from build123d import *

# Parameters (mm, degrees)
SKETCH1_W           = 300
SKETCH1_H           = 50
BOSS_EXTRUDE1_DEPTH = 6
SKETCH2_W           = 220
SKETCH2_H           = 25
CUT_EXTRUDE1_DEPTH  = 10
FILLET1_R           = 10


with BuildPart() as part:
    # Sketch1 → Boss-Extrude1 (new body)
    with BuildSketch(Plane(origin=(0, 0, 0), x_dir=(0, 0, -1), z_dir=(1, 0, 0))):
        Rectangle(SKETCH1_W, SKETCH1_H)
    extrude(amount=BOSS_EXTRUDE1_DEPTH)

    # Sketch2 → Cut-Extrude1 (cut)
    with BuildSketch(Plane(origin=(6, 0, 0), x_dir=(0, 0, -1), z_dir=(1, 0, 0))):
        with Locations((0, -12.5)):
            Rectangle(SKETCH2_W, SKETCH2_H)
    extrude(amount=-CUT_EXTRUDE1_DEPTH, mode=Mode.SUBTRACT)

    # Fillet1
    fillet1_edges = [part.edges().sort_by_distance(p)[0] for p in [
        (3, 0, 110),
        (3, 0, -110),
    ]]
    fillet(fillet1_edges, radius=FILLET1_R)


solid = part.part
Input: part model. Units: mm. Frame: model coordinates. A direction names the side the tool comes from. Coordinates: 2 decimals unless noted, no trailing zeros. Loops run counter-clockwise (first coordinate to the right, second up) from the corner with the lowest first, then second, coordinate; pieces in that order, holes last. Notation, with made-up numbers: (73, 41) -> (78, 41) arc R33 ccw to (78, 70) -> close; hole circle Ø10 at (-27.75, -35). An arc over 180 degrees is marked (long way). One line per item, written item: value.
(1) Draft query along Z for faces 1 (the face through (6, 6, 2)), 2 (the face through (3, 0, 150)), 3 (the face through (2.96, -3.01, -107.15)), 4 (the face through (3, 0, 1)). Return one class per face: pulls with the +Z half, pulls with the -Z half, needs draft (parallel to the pull), parting line crosses it, or undercut.
Answer below:
face 1: needs draft
face 2: pulls with the +Z half
face 3: undercut
face 4: undercut
(2) Cut plane D-D (y = -7). Output: boundary loops of the cut face in (x, z).
Answer below:
outline: (0, -150) -> (6, -150) -> (6, -109.54) -> (0, -109.54) -> close; (0, 109.54) -> (6, 109.54) -> (6, 150) -> (0, 150) -> close
(3) Set-up query: faces 5 (the face through (3, -25, -130)), 6 (the face through (3, -18, -110)). Return all of +Z, -Z, +X, -X, +Y, -Y with unobstructed straight access to the full face (end or side cutting, diameter ignored); none if empty.
Answer below:
face 5: +Z, -Z, +X, -X, -Y
face 6: +X, -X, -Y
(4) Cut plane A-A (y = -19.5). Output: boundary loops of the cut face in (x, z).
Answer below:
outline: (0, -150) -> (6, -150) -> (6, -110) -> (0, -110) -> close; (0, 110) -> (6, 110) -> (6, 150) -> (0, 150) -> close
(5) Cut plane C-C (z = 26.5). Output: boundary loops of the cut face in (x, y).
Answer below:
outline: (0, 0) -> (6, 0) -> (6, 25) -> (0, 25) -> close
(6) Cut plane B-B (x = 2.9). Output: boundary loops of the cut face in (y, z).
Answer below:
outline: (-25, -150) -> (25, -150) -> (25, 150) -> (-25, 150) -> (-25, 110) -> (-10, 110) arc R10 cw to (0, 100) -> (0, -100) arc R10 cw to (-10, -110) -> (-25, -110) -> close
(7) Ray query, line 1 along Z through (x, y) = (4.75, -12.5); line 2 along Y through (x, z) = (3.2, 88); line 3 along Z through (x, y) = (3.9, -6.5). Return the intervals inside material, ascending.
Answer below:
line 1: z = -150 to -110, 110 to 150
line 2: y = 0 to 25
line 3: z = -150 to -109.37, 109.37 to 150
